Geometry: final body of the model. Coordinates: model frame, mm. Give positions to 0.01 mm unless a question says otherwise; leave off trailing zeros. Write each loop counter-clockwise with the first axis right and the second up, starting at its lowest first coordinate (ties: lowest second). Pieces come first, ordered by that corner, then holes. Notation, with made-up numbers: M -31,64.25 L 20,64.25 A22 cw 20,101.25 Z; hole C -7.75,31.25 d4. An arc over 180 degrees is marked long. Use a Markdown table: item, result. Add a question column.
(1) Cut plane B-B (x = 0). Output: boundary loops of the cut face in (y, z), plus the area to 3 significant figures.
(2) Cut plane A-A (y = 64.5). Output: boundary loops of the cut face in (x, z), plus the area to 3 significant figures.
(3) Material intervals for L1, parallel to X at y = 95, z = 63.6; L2, parallel to X at y = 60, z = 52.9; L3, parallel to X at y = -60, z = 15.7, sorted ascending.
(4) Pin query (flat end, axial travel): pin 1 Ø2 at (x, y) = (45.5, -77) entering from +Z; pin 2 Ø8 at (x, y) = (-48.5, 3) entering from -Z; pin 3 Ø1.6 at (x, z) = (40.5, 18) entering from +Y. Return the tip coordinate at first contact, or that it passes through.
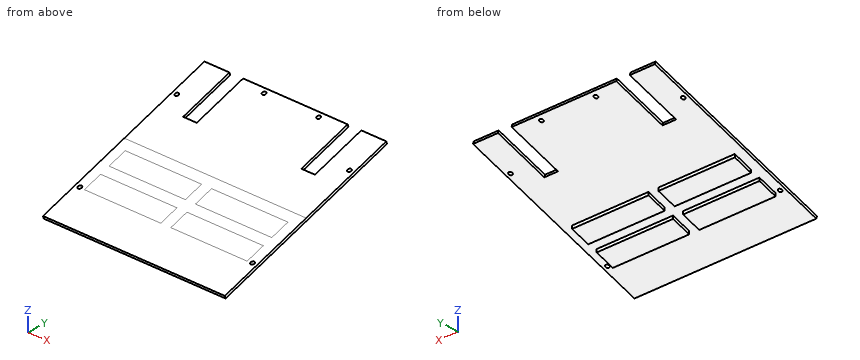
```python
from build123d import *

# Parameters (mm, degrees)
PAD032_DEPTH    = 3
SKETCH060_W     = 84
SKETCH060_H     = 20
PAD031_DEPTH    = 30
SKETCH062_R     = 2
POCKET023_DEPTH = 250
POCKET022_DEPTH = 250


with BuildPart() as part:
    # Sketch063 → Pad032 (new body)
    with BuildSketch(Plane(origin=(0, 0, 0), x_dir=(1, 0, 0), z_dir=(0, -0.292372, 0.956305))):
        Polygon((-100, 104.55), (-72.5, 104.55), (-72.5, 44.55), (-57.5, 44.55), (-57.5, 104.55), (57.5, 104.55), (57.5, 44.55), (72.5, 44.55), (72.5, 104.55), (100, 104.55), (100, -104.55), (-100, -104.55), align=None)
    extrude(amount=-PAD032_DEPTH)

    # Sketch060 → Pad031 (join, symmetric)
    with BuildSketch(Plane.XY):
        with Locations((-47.5, -50.5)):
            Rectangle(SKETCH060_W, SKETCH060_H)
        with Locations((47.5, -50.5)):
            Rectangle(SKETCH060_W, SKETCH060_H)
        with Locations((-47.5, -20)):
            Rectangle(SKETCH060_W, SKETCH060_H)
        with Locations((47.5, -20)):
            Rectangle(SKETCH060_W, SKETCH060_H)
    extrude(amount=PAD031_DEPTH, both=True)

    # Sketch062 → Pocket023 (cut, symmetric)
    with BuildSketch(Plane.XY):
        with Locations((-95, 60)):
            Circle(SKETCH062_R)
        with Locations((-95, -60)):
            Circle(SKETCH062_R)
        with Locations((95, -60)):
            Circle(SKETCH062_R)
        with Locations((95, 60)):
            Circle(SKETCH062_R)
        with Locations((-30, 95)):
            Circle(SKETCH062_R)
        with Locations((30, 95)):
            Circle(SKETCH062_R)
    extrude(amount=POCKET023_DEPTH, both=True, mode=Mode.SUBTRACT)

    # Sketch061 → Pocket022 (cut, symmetric)
    with BuildSketch(Plane.YZ):
        Polygon((-110, -33.630375), (130, 39.744989), (130, 89.744989), (-110, 16.369625), align=None)
        Polygon((-110, -40), (130, 33.375364), (130, -16.624636), (-110, -90), align=None)
    extrude(amount=POCKET022_DEPTH, both=True, mode=Mode.SUBTRACT)


with BuildPart() as part_1:
    # Body012 placement: moved
    add(part.part.moved(Location((0, 0, 36))))


solid = part_1.part
```
Answer list:
| question | item | result |
|---|---|---|
| 1 | outline | M -99.98,5.43 L -99.1,2.56 L 100.86,63.7 L 99.98,66.57 L 0.73,36.22 Z |
| 1 | area | 627 mm² |
| 2 | outline | M -100,52.58 L -72.5,52.58 L -72.5,55.72 L -100,55.72 Z; M -57.5,52.58 L 57.5,52.58 L 57.5,55.72 L -57.5,55.72 Z; M 72.5,52.58 L 100,52.58 L 100,55.72 L 72.5,55.72 Z |
| 2 | area | 533 mm² |
| 3 | L1 | -100 to -72.5, -57.5 to -32, -28 to 28, 32 to 57.5, 72.5 to 100 |
| 3 | L2 | -100 to -97, -93 to -72.5, -57.5 to 57.5, 72.5 to 93, 97 to 100 |
| 3 | L3 | -100 to -97, -93 to 93, 97 to 100 |
| 4 | pin 1 | z = 12.76 |
| 4 | pin 2 | z = 32.56 |
| 4 | pin 3 | y = -40.5 |
